Source: CAD feature listing. Evaluate the final solid. Frame: model axes, mm. Round coordinates to 2 decimals unless told otherwise and drop trailing zeros. Order: outer loops, then holes, each group sorted by start corner. A loop starts at its lowest first (then second) coordinate and runs counter-clockwise, first axis right, second up. Notation, with made-up numbers: (-25, 37) -> (11, 37) arc R8 cw to (11, 45) -> close; hole circle Ø4 at (-13, 15). An arc over 180 degrees is marked (long way). Answer as CSV lines item,"result". Start each with the question number.
(1) Section query B-B (y = -133.5). Output: boundary loops of the cut face in (x, z).
(2) Contact query for flat-ended pins moving along their axis: P1, Ø1.5, axis at y = -69, z = 2.5, coming from the +X side; P2, Ø8, axis at x = 11.5, y = 154, coming from the -Z side. Output: stop coordinate, or through.
(3) Line query: line 1 along X through (y, z) = (-52.5, 3.35); line 2 along Y through (x, z) = (60, 4.7); line 3 along Y through (x, z) = (-4.67, 2.6). Output: solid intervals per line, ascending. Write a range as from..to.
(4) Section query A-A (x = 45). Output: boundary loops of the cut face in (y, z).
(5) Section query C-C (x = 68.5). Output: boundary loops of the cut face in (y, z), plus the area to 3 significant figures.
(6) Section query D-D (z = 2.1). Count the separate pieces of the cut face and the enclosed holes in it, plus the area to 3 significant figures.
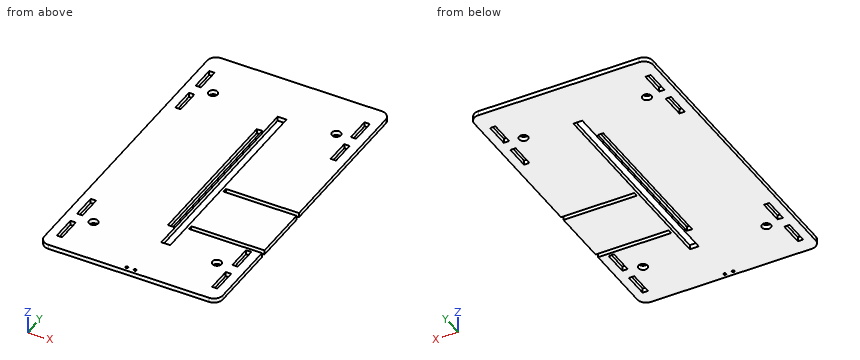
```python
from build123d import *

# Parameters (mm, degrees)
SKETCH1_R           = 5
BOSS_EXTRUDE1_DEPTH = 5
SKETCH4_W           = 6
SKETCH4_H           = 180
SKETCH4_W_2         = 10
SKETCH4_H_2         = 235.736115182
SKETCH4_W_3         = 82
SKETCH4_H_3         = 5
CUT_EXTRUDE1_DEPTH  = 10
SKETCH5_R           = 1.5
SKETCH5_W           = 6
SKETCH5_H           = 27.65
CUT_EXTRUDE2_DEPTH  = 6
FILLET1_R           = 10


with BuildPart() as part:
    # Sketch1 → Boss-Extrude1 (new body)
    with BuildSketch(Plane.XY):
        Polygon((100, 190), (-100, 190), (-100, -90), (-100, -160), (100, -160), (100, -90), align=None)
        with Locations((-69.105066414, 135.933866224)):
            Circle(SKETCH1_R, mode=Mode.SUBTRACT)
        with Locations((69.105066414, 135.933866224)):
            Circle(SKETCH1_R, mode=Mode.SUBTRACT)
        with Locations((69.105066414, -105.933866224)):
            Circle(SKETCH1_R, mode=Mode.SUBTRACT)
        with Locations((-69.105066414, -105.933866224)):
            Circle(SKETCH1_R, mode=Mode.SUBTRACT)
    extrude(amount=BOSS_EXTRUDE1_DEPTH)

    # Sketch4 → Cut-Extrude1 (cut)
    with BuildSketch(Plane.XY.offset(5)):
        with Locations((0, 15)):
            Rectangle(SKETCH4_W, SKETCH4_H)
        with Locations((10, 15)):
            Rectangle(SKETCH4_W_2, SKETCH4_H_2)
        with Locations((59, -68.15)):
            Rectangle(SKETCH4_W_3, SKETCH4_H_3)
        with Locations((59, 1.85)):
            Rectangle(SKETCH4_W_3, SKETCH4_H_3)
    extrude(amount=-CUT_EXTRUDE1_DEPTH, mode=Mode.SUBTRACT)

    # Sketch5 → Cut-Extrude2 (cut, through all)
    with BuildSketch(Plane.XY.offset(5)):
        with Locations((4.67, -155)):
            Circle(SKETCH5_R)
        with Locations((-4.67, -155)):
            Circle(SKETCH5_R)
        with Locations((-87, 152.175)):
            Rectangle(SKETCH5_W, SKETCH5_H)
        with Locations((-87, 111.115)):
            Rectangle(SKETCH5_W, SKETCH5_H)
        with Locations((-87, -87.845)):
            Rectangle(SKETCH5_W, SKETCH5_H)
        with Locations((-87, -128.905)):
            Rectangle(SKETCH5_W, SKETCH5_H)
        with Locations((87, -87.845)):
            Rectangle(SKETCH5_W, SKETCH5_H)
        with Locations((87, -128.905)):
            Rectangle(SKETCH5_W, SKETCH5_H)
        with Locations((87, 152.175)):
            Rectangle(SKETCH5_W, SKETCH5_H)
        with Locations((87, 111.115)):
            Rectangle(SKETCH5_W, SKETCH5_H)
    extrude(amount=-CUT_EXTRUDE2_DEPTH, mode=Mode.SUBTRACT)

    # Fillet1
    fillet1_edges = [part.edges().sort_by_distance(p)[0] for p in [
        (-100, 190, 2.5),
        (100, 190, 2.5),
        (100, -160, 2.5),
        (-100, -160, 2.5),
    ]]
    fillet(fillet1_edges, radius=FILLET1_R)


solid = part.part
```
Answer block:
1,outline,"(-100, 0) -> (-90, 0) -> (-90, 5) -> (-100, 5) -> close; (-84, 0) -> (84, 0) -> (84, 5) -> (-84, 5) -> close; (90, 0) -> (100, 0) -> (100, 5) -> (90, 5) -> close"
2,P1,"x = 18"
2,P2,"z = 0"
3,line 1,"-100..-3, 3..5, 15..100"
3,line 2,"-160..-70.65, -65.65..-0.65, 4.35..190"
3,line 3,"-160..-156.5, -153.5..190"
4,outline,"(-160, 0) -> (-70.65, 0) -> (-70.65, 5) -> (-160, 5) -> close; (-65.65, 0) -> (-0.65, 0) -> (-0.65, 5) -> (-65.65, 5) -> close; (4.35, 0) -> (190, 0) -> (190, 5) -> (4.35, 5) -> close"
5,outline,"(-160, 0) -> (-110.9, 0) -> (-110.9, 5) -> (-160, 5) -> close; (-100.97, 0) -> (-70.65, 0) -> (-70.65, 5) -> (-100.97, 5) -> close; (-65.65, 0) -> (-0.65, 0) -> (-0.65, 5) -> (-65.65, 5) -> close; (4.35, 0) -> (130.97, 0) -> (130.97, 5) -> (4.35, 5) -> close; (140.9, 0) -> (190, 0) -> (190, 5) -> (140.9, 5) -> close"
5,area,"1,600 mm2"
6,separate pieces,"1"
6,enclosed holes,"16"
6,area,"64,000 mm2"
